```python
from build123d import *

# Parameters (mm, degrees)
F1_DEPTH = 25.4
F2_DEPTH = 25.4
F3_W     = 15.985176
F3_H     = 10.561323
F4_DEPTH = 25.4


with BuildPart() as f1:
    # F0 (on Front) → F1 (new body)
    with BuildSketch(Plane.XZ):
        Polygon((0, 36.004499), (0, 0), (62.887855, 0), (62.887855, 36.004499), (46.902679, 36.004499), (46.902679, 12.330239), (16.79617, 12.330239), (16.79617, 36.004499), align=None)
    extrude(amount=F1_DEPTH)

    # F1_face (on face) → F2 (join)
    with BuildSketch(Plane(origin=(31.257644, -25.4, 15.170026), x_dir=(1, 0, 0), z_dir=(0, -1, 0))):
        Polygon((-31.257644, 20.834473), (-31.257644, -15.170026), (31.630211, -15.170026), (31.630211, 20.834473), (15.645035, 20.834473), (15.645035, -2.839787), (-14.461474, -2.839787), (-14.461474, 20.834473), align=None)
    extrude(amount=F2_DEPTH)

    # F3 (on face) → F4 (cut)
    with BuildSketch(Plane.XY.offset(36.004499)):
        with Locations((54.895267, -23.362921)):
            Rectangle(F3_W, F3_H)
    extrude(amount=-F4_DEPTH, mode=Mode.SUBTRACT)


solid = f1.part
```
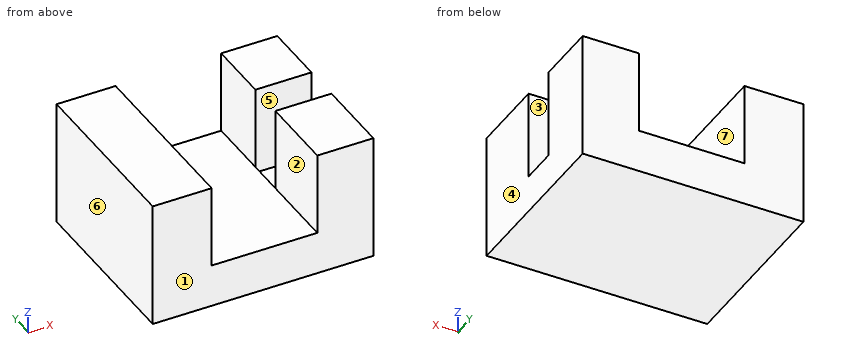
Verification items for the finished model (mm, model axes). Face numbers are marked on the shaded views. A direction names the side the tool comes from. Coordinates: 2 decimals unless noted, no trailing zeros. Loops run counter-clockwise (first coordinate to the right, second up) from the corner with the lowest first, then second, coordinate; pieces in that order, holes last. Notation, with made-up numbers: (-13.5, 49.5) - (27.5, 49.5) arc R17 cw to (27.5, 74.5) - close; hole circle Ø10 at (74, 3). An arc over 180 degrees is marked (long way). Return JSON: item names as keys, results as strings.
1. Section check C-C, the plane x = 50. Record the boundary of the cut face in (y, z), then the cut area to 3 significant figures.
Established:
{"outline": "(-50.8, 0) - (0, 0) - (0, 36) - (-18.08, 36) - (-18.08, 10.6) - (-28.64, 10.6) - (-28.64, 36) - (-50.8, 36) - close", "area": "1,560 mm2"}
2. Section check A-A, the plane z = 33. Record the boundary of the cut face in (x, y), then the cut area to 3 significant figures.
Established:
{"outline": "(0, -50.8) - (16.8, -50.8) - (16.8, 0) - (0, 0) - close; (46.9, -50.8) - (62.89, -50.8) - (62.89, -28.64) - (46.9, -28.64) - close; (46.9, -18.08) - (62.89, -18.08) - (62.89, 0) - (46.9, 0) - close", "area": "1,500 mm2"}
3. Mould release check, pull along X, two halves, no side actions. Record for the marked faces 4, 5, 6 and 7: +X half, -X half, draft (parallel to the pull), parting line (faces both ways), or undercut.
Established:
{"face 4": "+X half", "face 5": "draft", "face 6": "-X half", "face 7": "undercut"}
4. Section check D-D, the plane x = 24. Record the boundary of the cut face in (y, z), then the cut area to 3 significant figures.
Established:
{"outline": "(-50.8, 0) - (0, 0) - (0, 12.33) - (-50.8, 12.33) - close", "area": "626 mm2"}
5. Tool access check on the marked faces 1, 2 and 3. Record the directions out of +Z, -Z, +X, -X, +Y, -Y that give a thin tool (end or side, any length) a straight path to the whole face; none if there is none.
Established:
{"face 1": "+Z, -Z, +X, -X, -Y", "face 2": "+Z, +Y, -Y", "face 3": "+Z, +X"}
6. Section check B-B, the plane y = -21. Record the boundary of the cut face in (x, z), then the cut area to 3 significant figures.
Established:
{"outline": "(0, 0) - (62.89, 0) - (62.89, 10.6) - (46.9, 10.6) - (46.9, 12.33) - (16.8, 12.33) - (16.8, 36) - (0, 36) - close", "area": "1,150 mm2"}
7. Go/stop test with flat-tipped pins: pin 1 (5.5 mm diameter, centred on x = 51, y = -24, fed in from +Z); pin 2 (0.5 mm diameter, centred on y = -21, z = 11, fed in from +X); pin 3 (9 mm diameter, centred on x = 25, y = -26, fed in from +Z). Record where each tip stops, or that it passes through.
Established:
{"pin 1": "stops at z = 10.6", "pin 2": "stops at x = 46.9", "pin 3": "stops at z = 12.33"}
8. Thickness scan on L1, parallel to X at y = -33.5, z = 31; L2, parallel to Y at x = 47.5, z = 14; L3, parallel to X at y = -27.5, z = 30.5. Record the ranges inside material, lowest first.
Established:
{"L1": "x = 0 to 16.8, 46.9 to 62.89", "L2": "y = -50.8 to -28.64, -18.08 to 0", "L3": "x = 0 to 16.8"}
